Part model, mm, in its own coordinate system. Give positions to 0.01 mm unless a question says otherwise; leave off trailing zeros. Order: outer loops, then holes, each group sorted by start corner. A loop starts at its lowest first (then second) coordinate and runs counter-clockwise, first axis right, second up. Notation, with made-up numbers: M 66.5,53 L 91.5,53 A28 cw 91.5,79 Z; hole C 22,47.25 d2. An arc over 180 degrees is marked long. Return JSON: item names as keys, results as strings.
from build123d import *

# Parameters (mm, degrees)
ESQUISSE1_R                  = 16
ESQUISSE1_R_2                = 13
BOSS_EXTRU_1_DEPTH           = 900
ENL_V_MAT_EXTRU_1_DEPTH      = 901.284399509
ENL_V_MAT_EXTRU_1_DEPTH_BACK = 901.284399509
ENL_V_MAT_EXTRU_2_DEPTH      = 901.284399509
ENL_V_MAT_EXTRU_2_DEPTH_BACK = 901.284399509


with BuildPart() as part:
    # Esquisse1 → Boss.-Extru.1 (new body)
    with BuildSketch(Plane.XY):
        Circle(ESQUISSE1_R)
        Circle(ESQUISSE1_R_2, mode=Mode.SUBTRACT)
    extrude(amount=BOSS_EXTRU_1_DEPTH)

    # Esquisse2 → Enlèv. mat.-Extru.1 (cut, two sides: drawn at the far end of the back side and taken through both)
    with BuildSketch(Plane(origin=(0, 0, 0), x_dir=(1, 0, 0), z_dir=(0, 1, 0)).offset(-ENL_V_MAT_EXTRU_1_DEPTH_BACK)):
        Polygon((0, 0), (16, -100), (16, 0), align=None)
    extrude(amount=ENL_V_MAT_EXTRU_1_DEPTH + ENL_V_MAT_EXTRU_1_DEPTH_BACK, mode=Mode.SUBTRACT)

    # Esquisse3 → Enlèv. mat.-Extru.2 (cut, two sides: drawn at the far end of the back side and taken through both)
    with BuildSketch(Plane(origin=(0, 0, 0), x_dir=(1, 0, 0), z_dir=(0, 1, 0)).offset(-ENL_V_MAT_EXTRU_2_DEPTH_BACK)):
        Polygon((0, 0), (-16, -100), (-16, 0), align=None)
    extrude(amount=ENL_V_MAT_EXTRU_2_DEPTH + ENL_V_MAT_EXTRU_2_DEPTH_BACK, mode=Mode.SUBTRACT)


solid = part.part
Q1. Band-saw the part on A-A (y = 0). Give the cut face in (x, z).
Established:
{"outline": "M -16,100 L -13,81.25 L -13,900 L -16,900 Z; M 13,81.25 L 16,100 L 16,900 L 13,900 Z"}
Q2. Band-saw the part on B-B (z = 168). Give the cut face in (x, y), then the cut area to 3 significant figures.
Established:
{"outline": "C 0,0 d32; hole C 0,0 d26", "area": "273 mm²"}
Q3. Probe line 1 along X through (y, z) = (-1, 525); line 2 along Y through (x, z) = (0, 266.5); line 3 along Y through (x, z) = (-4, 139). List the from-to ranges inside material, lowest first.
Established:
{"line 1": "x = -15.97 to -12.96, 12.96 to 15.97", "line 2": "y = -16 to -13, 13 to 16", "line 3": "y = -15.49 to -12.37, 12.37 to 15.49"}
Q4. Pin check, flat tips, straight feed: pin 1 (6 mm diameter, centred on y = -4.5, z = 293.5, fed in from +X); pin 2 (3 mm diameter, centred on y = -2.5, z = 438.5, fed in from +X); pin 3 (8 mm diameter, centred on x = 7.5, z = 201, fed in from -Y); pin 4 (12 mm diameter, centred on x = 4.5, y = -4, fed in from +Z). Stop position of each tip, or through.
Established:
{"pin 1": "stops at x = 15.93", "pin 2": "stops at x = 15.97", "pin 3": "stops at y = -15.61", "pin 4": "passes through"}
